from build123d import *

# Parameters (mm, degrees)
SKETCH_1_R           = 1.75
EXTRUDE_1_DEPTH      = 10
FILLET_8_R           = 5
CUT_EXTRUDE_7_DEPTH  = 2.5
CUT_EXTRUDE_8_DEPTH  = 2.5
CUT_EXTRUDE_9_DEPTH  = 5
FILLET_10_R          = 5
SKETCH_12_R          = 2.5
CUT_EXTRUDE_10_DEPTH = 10


with BuildPart() as part:
    # 스케치1 → 보스-돌출1 (new body)
    with BuildSketch(Plane.XY):
        Polygon((-6.904227126, 6.544293027), (-22.050718655, -0.000460165), (-16.973385404, -11.96794474), (-4.104227126, -6.455706973), (23.095772874, -6.455706973), (23.095772874, 6.544293027), align=None)
        with Locations((-16.323899965, -4.537411593)):
            Circle(SKETCH_1_R, mode=Mode.SUBTRACT)
        with Locations((19.595772874, 0.044293027)):
            Circle(SKETCH_1_R, mode=Mode.SUBTRACT)
    extrude(amount=EXTRUDE_1_DEPTH)

    # 필렛8
    fillet_8_edges = [part.edges().sort_by_distance(p)[0] for p in [
        (23.095772874, -6.455706973, 5),
        (-4.104227126, -6.455706973, 5),
        (-16.973385404, -11.96794474, 5),
        (-22.050718655, -0.000460165, 5),
        (-6.904227126, 6.544293027, 5),
        (23.095772874, 6.544293027, 5),
    ]]
    fillet(fillet_8_edges, radius=FILLET_8_R)

    # 스케치9 → 컷-돌출7 (cut)
    with BuildSketch(Plane.XY.offset(5)):
        Polygon((-22.050718655, -0.000460165), (-6.904227126, 6.544293027), (-4.104227126, -6.455706973), (-16.973385404, -11.96794474), align=None)
    extrude(amount=-CUT_EXTRUDE_7_DEPTH, mode=Mode.SUBTRACT)

    # 스케치10 → 컷-돌출8 (cut)
    with BuildSketch(Plane.XY.offset(5)):
        Polygon((-22.050718655, -0.000460165), (-6.904227126, 6.544293027), (-4.104227126, -6.455706973), (-16.973385404, -11.96794474), align=None)
    extrude(amount=CUT_EXTRUDE_8_DEPTH, mode=Mode.SUBTRACT)

    # 스케치11 → 컷-돌출9 (cut)
    with BuildSketch(Plane.XY.offset(5)):
        Polygon((8.095772874, 6.544293027), (23.109867502, 6.568608602), (23.095772874, -6.455706973), (8.095772874, -6.455706973), align=None)
    extrude(amount=-CUT_EXTRUDE_9_DEPTH, mode=Mode.SUBTRACT)

    # 필렛10
    fillet_10_edges = [part.edges().sort_by_distance(p)[0] for p in [
        (8.095772874, 0.044293027, 0),
    ]]
    fillet(fillet_10_edges, radius=FILLET_10_R - 0.0001)  # a hair under: the kernel refuses the full size

    # 스케치12 → 컷-돌출10 (cut)
    with BuildSketch(Plane(origin=(0, 6.544293027, 0), x_dir=(1, 0, 0), z_dir=(0, 1, 0))):
        with Locations(Location((1.29393204, -5, 0), (0, 0, 270))):
            Circle(SKETCH_12_R)
    extrude(amount=-CUT_EXTRUDE_10_DEPTH, mode=Mode.SUBTRACT)


solid = part.part
For this review, take the finished solid that the model builds, in its own axes (mm). A direction names the side the tool comes from. Give positions to 0.01 mm unless a question says otherwise; leave off trailing zeros. Loops run counter-clockwise (first coordinate to the right, second up) from the corner with the lowest first, then second, coordinate; pieces in that order, holes last. Notation, with made-up numbers: M 13.25,41.5 L 57.25,41.5 A23 ccw 57.25,64.5 Z; hole C 13.25,-25 d5. An arc over 180 degrees is marked long. Answer as a JSON object with one key per item and string values. Group by question number.
Q1. Add section C-C on z = 5.75. Give the boundary of the cut face in (x, y), and give its area (3 significant figures).
Q2. Tool access review of faces 4 (the flat face through (16, 0, 5)), 5 (the flat face through (-8.76, -8.45, 1.23)), 6 (the cylindrical face through (2, 1.6, 7.4)): name each direction out of +Z, -Z, +X, -X, +Y, -Y from which nothing blocks a thin tool from reaching the whole face with its end or side.
Q3. Add section A-A on x = 20.5. Give the boundary of the cut face in (y, z).
Q4. Mouldability with a two-part tool opening along Y and no side actions: class faces 1 (the flat face through (1, -3.456, 5)), 2 (the flat face through (5, -6.456, 6)), 3 (the cylindrical face through (21, -1, 7)) as +Y half, -Y half, draft (parallel to the pull), parting line (faces both ways), or undercut.
Q5. Add section B-B on y = -8.75. Give the boundary of the cut face in (x, z).
Q6. Insertion check: P1, Ø2, axis at x = -16.32, y = -4.54, coming from the -Z side; P2, Ø6, axis at y = -7, z = 5, coming from the -X side; P3, Ø4, axis at x = 19.6, y = 0.04, coming from the +Z side; P4, Ø6.5, axis at x = 19, y = -2.5, coming from the -Z side. Each pin has a flat end and moves straight along its axis. Give the tip position at first contact, or say it passes through.
Q7. For probe 1 along Z at (x, y) = (-11.5, -6.5); probe 2 along Z at (x, y) = (15, 5.5); probe 3 along Y at (x, z) = (1, 8), list the stretches that pass through material, from the lowest coordinate up. Write a range as [from, to].
Q8. Add section D-D on y = -5. Give the number of separate pieces and of enclosed holes in the cut face, and give its area (3 significant figures).
Checked values:
{
 "1": {"outline": "M -6.88,6.44 L -4.1,-6.46 L -5.05,-6.86 A5 cw -3.08,-6.46 L 18.1,-6.46 A5 ccw 23.1,-1.46 L 23.1,1.54 A5 ccw 18.1,6.54 L 3.68,6.54 L 3.68,-3.46 L -1.09,-3.46 L -1.09,6.54 L -5.87,6.54 A5 ccw Z; hole C 19.6,0.04 d3.5", "area": "304 mm²"},
 "2": {"face 4": "-Z, +X, +Y, -Y", "face 5": "+Z, -Z, +X, -Y", "face 6": "+Y"},
 "3": {"outline": "M -5.84,5 L -1.45,5 L -1.45,10 L -5.84,10 Z; M 1.54,5 L 5.93,5 L 5.93,10 L 1.54,10 Z"},
 "4": {"face 1": "+Y half", "face 2": "-Y half", "face 3": "undercut"},
 "5": {"outline": "M -18.04,0 L -9.46,0 L -9.46,2.5 L -18.04,2.5 Z; M -18.04,7.5 L -9.46,7.5 L -9.46,10 L -18.04,10 Z"},
 "6": {"P1": "through", "P2": "x = -19.78", "P3": "z = 10", "P4": "z = 5"},
 "7": {"probe 1": "[0, 2.5], [7.5, 10]", "probe 2": "[5, 10]", "probe 3": "[-6.46, 6.54]"},
 "8": {"separate pieces": "3", "enclosed holes": "0", "area": "248 mm²"}
}
